Verification items for the finished model (mm, model axes). Give positions to 0.01 mm unless a question says otherwise; leave off trailing zeros. Write each loop counter-clockwise with the first axis right and the second up, starting at its lowest first coordinate (ties: lowest second). Pieces come first, ordered by that corner, then holes. Notation, with made-up numbers: (75.25, 29) - (125.25, 29) arc R25 ccw to (125.25, 59) - close; hole circle Ø11 at (80, 22). An arc over 180 degrees is marked (long way). Put each result on its own line as item: value.
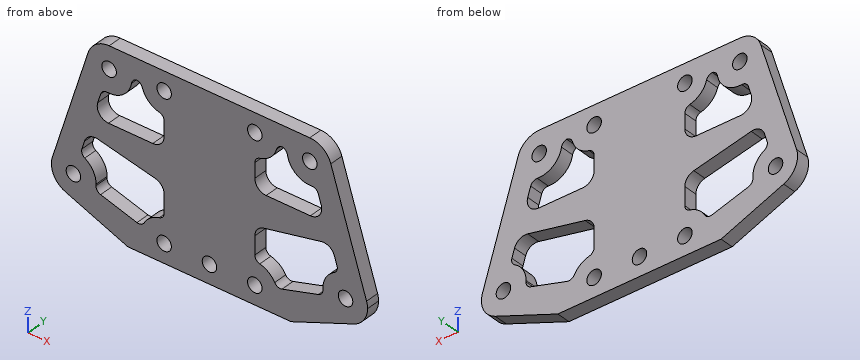
from build123d import *

# Parameters (mm, degrees)
SKETCH_1_R             = 1.6
EXTRUDE_1_DEPTH        = 3
SKETCH_2_R             = 1.6
CUT_EXTRUDE_1_DEPTH    = 59.077534383
CUT_EXTRUDE_2_DEPTH    = 10
CUT_EXTRUDE_3_DEPTH    = 10
FILLET_1_R             = 2.5
FILLET_2_R             = 1.4
FILLET_1_OF_MIRROR_1_R = 2.5
FILLET_2_OF_MIRROR_1_R = 1.4


with BuildPart() as part:
    # 草图1 → 凸台-拉伸1 (new body)
    with BuildSketch(Plane(origin=(0, 0, 0), x_dir=(1, 0, 0), z_dir=(0, 1, 0))):
        Polygon((42, 0), (-42, 0), (-42, 40), (0, 40), (42, 40), align=None)
        with Locations(Location((-22.12, 4.86, 0), (0, 0, 270))):
            Circle(SKETCH_1_R, mode=Mode.SUBTRACT)
        with Locations(Location((-30, 30, 0), (0, 0, 270))):
            Circle(SKETCH_1_R, mode=Mode.SUBTRACT)
        with Locations(Location((30, 30, 0), (0, 0, 90))):
            Circle(SKETCH_1_R, mode=Mode.SUBTRACT)
        with Locations(Location((22.12, 4.86, 0), (0, 0, 90))):
            Circle(SKETCH_1_R, mode=Mode.SUBTRACT)
    extrude(amount=EXTRUDE_1_DEPTH)

    # 草图2 → 切除-拉伸1 (cut, through all)
    with BuildSketch(Plane(origin=(0, 3, 0), x_dir=(1, 0, 0), z_dir=(0, 1, 0))):
        with Locations(Location((-10, 35.85, 0), (0, 0, 270))):
            Circle(SKETCH_2_R)
        with Locations(Location((10, 35.85, 0), (0, 0, 270))):
            Circle(SKETCH_2_R)
        with Locations(Location((-10, 4.15, 0), (0, 0, 270))):
            Circle(SKETCH_2_R)
        with Locations(Location((10, 4.15, 0), (0, 0, 270))):
            Circle(SKETCH_2_R)
        with Locations(Location((0, 35.85, 0), (0, 0, 270))):
            Circle(SKETCH_2_R)
    extrude(amount=-CUT_EXTRUDE_1_DEPTH, mode=Mode.SUBTRACT)

    # 草图3 → 切除-拉伸2 (cut)
    with BuildSketch(Plane(origin=(0, 3, 0), x_dir=(1, 0, 0), z_dir=(0, 1, 0))):
        with BuildLine():
            ThreePointArc((-22.12, 0), (-24.997070445, 0.943105101), (-26.757523684, 3.406392735))
            Line((-26.757523684, 3.406392735), (-34.637523684, 28.546392735))
            ThreePointArc((-34.637523684, 28.546392735), (-34.388052817, 32.089160711), (-31.795255063, 34.516266075))
            Line((-31.795255063, 34.516266075), (-18, 40))
            Line((-18, 40), (-42, 40))
            Line((-42, 40), (-42, 0))
            Line((-42, 0), (-22.12, 0))
        make_face()
        with BuildLine():
            ThreePointArc((26.757523684, 3.406392735), (24.997070445, 0.943105101), (22.12, 0))
            Line((22.12, 0), (42, 0))
            Line((42, 0), (42, 40))
            Line((42, 40), (18, 40))
            Line((18, 40), (31.795255063, 34.516266075))
            ThreePointArc((31.795255063, 34.516266075), (34.021476073, 32.728979699), (34.86, 30))
            ThreePointArc((34.86, 30), (34.804058966, 29.264733077), (34.637523684, 28.546392735))
            Line((34.637523684, 28.546392735), (26.757523684, 3.406392735))
        make_face()
    extrude(amount=-CUT_EXTRUDE_2_DEPTH, mode=Mode.SUBTRACT)

    # 草图4 → 切除-拉伸3 (cut)
    with BuildSketch(Plane(origin=(0, 3, 0), x_dir=(1, 0, 0), z_dir=(0, 1, 0))):
        with BuildLine():
            Line((-14.798923626, 34.446314839), (-25.201076374, 31.403685161))
            ThreePointArc((-25.201076374, 31.403685161), (-25.050524365, 30.709007006), (-25, 30))
            ThreePointArc((-25, 30), (-25.970272737, 27.040050982), (-28.504519275, 25.228885099))
            Line((-28.504519275, 25.228885099), (-26.865552904, 20))
            Line((-26.865552904, 20), (-10, 23.584883936))
            Line((-10, 23.584883936), (-10, 30.85))
            ThreePointArc((-10, 30.85), (-12.998464123, 31.848848553), (-14.798923626, 34.446314839))
        make_face()
        with BuildLine():
            Line((-10, 16.15), (-25.658790772, 16.15))
            Line((-25.658790772, 16.15), (-23.615480725, 9.631114901))
            ThreePointArc((-23.615480725, 9.631114901), (-19.160050982, 8.889727263), (-17.12, 4.86))
            ThreePointArc((-17.12, 4.86), (-17.122139776, 4.713735907), (-17.128557274, 4.567597002))
            Line((-17.128557274, 4.567597002), (-14.991442726, 4.442402998))
            ThreePointArc((-14.991442726, 4.442402998), (-13.430596523, 7.787445188), (-10, 9.15))
            Line((-10, 9.15), (-10, 16.15))
        make_face()
    cut_extrude_3 = extrude(amount=-CUT_EXTRUDE_3_DEPTH, mode=Mode.SUBTRACT)

    # 圆角1
    fillet_1_edges = [part.edges().sort_by_distance(p)[0] for p in [
        (-10, 1.5, -23.584883936),
        (-26.865552904, 1.5, -20),
        (-25.658790772, 1.5, -16.15),
        (-10, 1.5, -16.15),
    ]]
    fillet(fillet_1_edges, radius=FILLET_1_R)

    # 圆角2
    # the kernel refuses this fillet: 1.4 mm, written as the material it adds along each edge
    with BuildSketch(Plane(origin=(-23.615480725, 3, -9.631114901), x_dir=(0.9813413175629745, 0, -0.1922738111230053), z_dir=(0, -1, 0)), Plane(origin=(-14.991442726, 3, -4.442402998), x_dir=(0.1679804165145185, 0, -0.9857903325086977), z_dir=(0, -1, 0))) as fillet_2_piece_1:
        with BuildLine():
            CenterArc((1.254493801, -1.391497509), FILLET_2_R, 96.317812547, 77.364374907)
            Line((-0.137003708, -1.237436867), (0, 0))
            ThreePointArc((0, 0), (0.55021658, -0.030366038), (1.100433159, 0))
        make_face()
    extrude(amount=3)
    with BuildSketch(Plane(origin=(-10, 3, -9.15), x_dir=(0, 0, -1), z_dir=(0, -1, 0)), Plane(origin=(-17.128557274, 3, -4.567597002), x_dir=(0.998288545196741, 0, 0.058480599594858615), z_dir=(0, -1, 0))) as fillet_2_piece_2:
        with BuildLine():
            CenterArc((1.244997998, -1.4), FILLET_2_R, 90, 77.364374907)
            ThreePointArc((-0.121095314, -1.09375), (-0.030366038, -0.55021658), (0, 0))
            Line((0, 0), (1.244997998, 0))
        make_face()
    extrude(amount=3)
    with BuildSketch(Plane(origin=(-10, 3, -30.85), x_dir=(0, 0, 1), z_dir=(0, -1, 0)), Plane(origin=(-25.201076374, 3, -31.403685161), x_dir=(0.9597847252329514, 0, -0.2807370321306184), z_dir=(0, -1, 0))) as fillet_2_piece_3:
        with BuildLine():
            CenterArc((1.244997998, 1.4), FILLET_2_R, 192.635625093, 77.364374907)
            ThreePointArc((-0.121095314, 1.09375), (-0.030366038, 0.55021658), (0, 0))
            Line((0, 0), (1.244997998, 0))
        make_face()
    extrude(amount=3)
    with BuildSketch(Plane(origin=(-14.798923626, 3, -34.446314839), x_dir=(0.3846499515684246, 0, 0.9230625194202224), z_dir=(0, -1, 0)), Plane(origin=(-28.504519275, 3, -25.228885099), x_dir=(0.9155142544303774, 0, -0.4022855328430172), z_dir=(0, -1, 0))) as fillet_2_piece_4:
        with BuildLine():
            CenterArc((1.254493801, 1.391497509), FILLET_2_R, 186.317812547, 77.364374907)
            Line((-0.137003708, 1.237436867), (0, 0))
            ThreePointArc((0, 0), (0.55021658, 0.030366038), (1.100433159, 0))
        make_face()
    extrude(amount=3)

    # 镜向1: 切除-拉伸3 across plane
    add(cut_extrude_3.mirror(Plane(origin=(0, 0, 0), x_dir=(0, 0, 1), z_dir=(1, 0, 0))), mode=Mode.SUBTRACT)

    # 圆角1 of 镜向1
    fillet_1_of_mirror_1_edges = [part.edges().sort_by_distance(p)[0] for p in [
        (10, 1.5, -23.584883936),
        (26.865552904, 1.5, -20),
        (25.658790772, 1.5, -16.15),
        (10, 1.5, -16.15),
    ]]
    fillet(fillet_1_of_mirror_1_edges, radius=FILLET_1_OF_MIRROR_1_R)

    # 圆角2 of 镜向1
    # the kernel refuses this fillet: 1.4 mm, written as the material it adds along each edge
    with BuildSketch(Plane(origin=(23.615480725, 3, -9.631114901), x_dir=(0.2990961449676297, 0, -0.9542229802648344), z_dir=(0, -1, 0)), Plane(origin=(10, 3, -30.85), x_dir=(0, 0, 1), z_dir=(0, -1, 0)), Plane(origin=(25.201076374, 3, -31.403685161), x_dir=(-0.9597847252329514, 0, -0.2807370321306184), z_dir=(0, -1, 0)), Plane(origin=(14.991442726, 3, -4.442402998), x_dir=(0.9982885451967423, 0, -0.05848059959483981), z_dir=(0, -1, 0))) as fillet_2_of_mirror_1_piece_1:
        with BuildLine():
            CenterArc((1.244997998, -1.4), FILLET_2_OF_MIRROR_1_R, 90, 77.364374907)
            ThreePointArc((-0.121095314, -1.09375), (-0.030366038, -0.55021658), (0, 0))
            Line((0, 0), (1.244997998, 0))
        make_face()
    extrude(amount=3)
    with BuildSketch(Plane(origin=(10, 3, -9.15), x_dir=(0.993926792387083, 0, 0.11004331590389448), z_dir=(0, -1, 0)), Plane(origin=(14.798923626, 3, -34.446314839), x_dir=(-0.3846499515684246, 0, 0.9230625194202224), z_dir=(0, -1, 0)), Plane(origin=(28.504519275, 3, -25.228885099), x_dir=(-0.9155142544303774, 0, -0.4022855328430172), z_dir=(0, -1, 0)), Plane(origin=(17.128557274, 3, -4.567597002), x_dir=(0.05172954697013894, 0, -0.9986611306996304), z_dir=(0, -1, 0))) as fillet_2_of_mirror_1_piece_2:
        with BuildLine():
            CenterArc((1.254493801, -1.391497509), FILLET_2_OF_MIRROR_1_R, 96.317812547, 77.364374907)
            Line((-0.137003708, -1.237436867), (0, 0))
            ThreePointArc((0, 0), (0.55021658, -0.030366038), (1.100433159, 0))
        make_face()
    extrude(amount=3)


solid = part.part
Q1. Section check C-C, the plane y = 0.85. Give the number of separate pieces and of enclosed holes in the cut face, plus the area to 3 significant figures.
Answers follow:
separate pieces: 1
enclosed holes: 13
area: 1,750 mm2
Q2. Section check A-A, the plane x = 0. Record the cut outline in (y, z), plus the area to 3 significant figures.
Answers follow:
outline: (0, -40) - (3, -40) - (3, -37.45) - (0, -37.45) - close; (0, -34.25) - (3, -34.25) - (3, 0) - (0, 0) - close
area: 110 mm2
Q3. Section check B-B, the plane x = -30. Record the cut outline in (y, z).
Answers follow:
outline: (0, -35.23) - (3, -35.23) - (3, -31.6) - (0, -31.6) - close; (0, -28.4) - (3, -28.4) - (3, -13.75) - (0, -13.75) - close
Q4. Scan lines: line 1 along X through (y, z) = (0.6, -30); line 2 along X through (y, z) = (1.8, -4.15); line 3 along Z through (x, y) = (13, 1.1). Record each from-to range of solid material in increasing order.
Answers follow:
line 1: x = -34.86 to -31.6, -28.4 to -25, -10.06 to 10.06, 25 to 28.4, 31.6 to 34.86
line 2: x = -26.99 to -23.55, -20.69 to -11.6, -8.4 to 8.4, 11.6 to 20.69, 23.55 to 26.99
line 3: z = -40 to -31.85, -22.95 to -16.15, -8.15 to 0
Q5. Go/stop test with flat-tipped pins: pin 1 Ø1 at (x, y) = (-26, 0.5) entering from -Z; pin 2 Ø1 at (y, z) = (0.5, -7.5) entering from +X. Record where each tip stops, or that it passes through.
Answers follow:
pin 1: stops at z = -37.02
pin 2: stops at x = 28.2
